from build123d import *

# Parameters (mm, degrees)
SKETCH1_R               = 10
BOSS_EXTRUDE1_DEPTH     = 30
F_5_0MM_DOWEL_HOLE1_D   = 5
SALIENTE_EXTRUIR1_START = 20
SALIENTE_EXTRUIR1_DEPTH = 20


with BuildPart() as part:
    # Sketch1 → Boss-Extrude1 (new body)
    with BuildSketch(Plane(origin=(0, 0, 0), x_dir=(1, 0, 0), z_dir=(0, 1, 0))):
        with Locations(Location((0, 0, 0), (0, 0, 270))):
            Circle(SKETCH1_R)
    extrude(amount=BOSS_EXTRUDE1_DEPTH)

    # Ø5.0mm Dowel Hole1 (through all)
    with Locations(Plane(origin=(0, 30, 0), x_dir=(1, 0, 0), z_dir=(0, 1, 0))):
        with Locations((0, 0)):
            Hole(F_5_0MM_DOWEL_HOLE1_D / 2)

    # Croquis1 → Saliente-Extruir1 (add)
    with BuildSketch(Plane.XZ.offset(SALIENTE_EXTRUIR1_START)):
        with BuildLine():
            Line((9.659258263, -2.588190451), (-2.588190451, 9.659258263))
            ThreePointArc((-2.588190451, 9.659258263), (7.071067812, 7.071067812), (9.659258263, -2.588190451))
        make_face()
    extrude(amount=-SALIENTE_EXTRUIR1_DEPTH)


solid = part.part
Design review of the part built by this model. Coordinates are the model's own, in mm. Give positions to 0.01 mm unless a question says otherwise; leave off trailing zeros. Loops run counter-clockwise (first coordinate to the right, second up) from the corner with the lowest first, then second, coordinate; pieces in that order, holes last. Notation, with made-up numbers: (19.25, -22) - (76.25, -22) arc R27 cw to (76.25, 2) - close; hole circle Ø10 at (9, -9.75). An arc over 180 degrees is marked (long way). Write item = value, one per line.
1) Take a section at C-C on x = 3.25. State the section outline as (y, z) points, and give its area (3 significant figures).
Result sheet:
outline = (-20, 3.82) - (0, 3.82) - (0, -9.46) - (30, -9.46) - (30, 9.46) - (-20, 9.46) - close
area = 680 mm2
2) Take a section at D-D on z = 6.5. State the section outline as (x, y) points.
Result sheet:
outline = (-7.6, 0) - (0.57, 0) - (0.57, -20) - (7.6, -20) - (7.6, 30) - (-7.6, 30) - close
3) Clearance check with flat-ended pins moving along their axes: pin 1 Ø3 at (x, y) = (2, 16) entering from -Z; pin 2 Ø1.5 at (x, y) = (-4.5, 18) entering from +Z; pin 3 Ø4 at (x, z) = (-4.5, -4.5) entering from -Y. State where each tip first meets the part, or that it passes through.
Result sheet:
pin_1 = -9.99
pin_2 = 9.27
pin_3 = 0
4) Take a section at A-A on z = -1.25. State the section outline as (x, y) points.
Result sheet:
outline = (-9.92, 0) - (-2.17, 0) - (-2.17, 30) - (-9.92, 30) - close; (2.17, 0) - (8.32, 0) - (8.32, -20) - (9.92, -20) - (9.92, 30) - (2.17, 30) - close
5) To check wall thickness, follow line 1 (Z direction, x = 0, y = 7.25); line 2 (Z direction, x = 1, y = 1); line 3 (Y direction, x = -3.25, z = 1.5). State the ranges of each line that lie inside material, in increasing order.
Result sheet:
line_1 = -10 to -2.5, 2.5 to 10
line_2 = -9.95 to -2.29, 2.29 to 9.95
line_3 = 0 to 30
6) Take a section at B-B on x = 0. State the section outline as (y, z) points.
Result sheet:
outline = (-20, 7.07) - (0, 7.07) - (0, 2.5) - (30, 2.5) - (30, 10) - (-20, 10) - close; (0, -10) - (30, -10) - (30, -2.5) - (0, -2.5) - close
7) Draft analysis for pull direction X (two halves, no side actions). For faces 1 (the face through (3.62, -10.14, 3.45)), 2 (the face through (0.54, 14.79, 2.44)), 3 (the face through (-2, 0, -2)), state which applies: +X half, -X half, draft (parallel to the pull), parting line (faces both ways), or undercut.
Result sheet:
face_1 = -X half
face_2 = undercut
face_3 = draft
